Here's how the part is built. I have some questions about the finished solid (model axes, mm). Face numbers are marked on the shaded views. A direction names the side the tool comes from. Round coordinates to 2 decimals unless told otherwise and drop trailing zeros. Order: outer loops, then holes, each group sorted by start corner. A loop starts at its lowest first (then second) coordinate and runs counter-clockwise, first axis right, second up. Notation, with made-up numbers: (41, 41.5) - (62, 41.5) arc R31 cw to (62, 69.5) - close; hole circle Ø10 at (35, -28). An arc over 180 degrees is marked (long way). Answer as a JSON object with one key per item and string values.
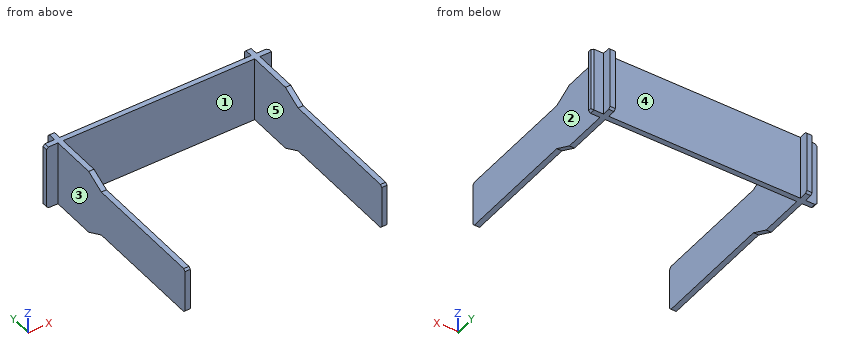
```python
from build123d import *

# Parameters (mm, degrees)
SKETCH1_W           = 2.75
SKETCH1_H           = 5
SKETCH1_W_2         = 6
SKETCH1_H_2         = 2.75
SKETCH1_H_3         = 98.25
SKETCH1_W_3         = 100.5
BOSS_EXTRUDE1_DEPTH = 17
CUT_EXTRUDE1_DEPTH  = 113
CHAMFER1_SIZE       = 1


with BuildPart() as part:
    # Sketch1 → Boss-Extrude1 (new body, symmetric)
    with BuildSketch(Plane.XY):
        with Locations((-51.625, 3.875)):
            Rectangle(SKETCH1_W, SKETCH1_H)
        with Locations((-56, 0)):
            Rectangle(SKETCH1_W_2, SKETCH1_H_2)
        with Locations((-51.625, 0)):
            Rectangle(SKETCH1_W, SKETCH1_H_2)
        with Locations((-51.625, -50.5)):
            Rectangle(SKETCH1_W, SKETCH1_H_3)
        Rectangle(SKETCH1_W_3, SKETCH1_H_2)
        with Locations((51.625, 3.875)):
            Rectangle(SKETCH1_W, SKETCH1_H)
        with Locations((51.625, 0)):
            Rectangle(SKETCH1_W, SKETCH1_H_2)
        with Locations((56, 0)):
            Rectangle(SKETCH1_W_2, SKETCH1_H_2)
        with Locations((51.625, -50.5)):
            Rectangle(SKETCH1_W, SKETCH1_H_3)
    extrude(amount=BOSS_EXTRUDE1_DEPTH, both=True)

    # Sketch2 → Cut-Extrude1 (cut, through all)
    with BuildSketch(Plane(origin=(53, 0, 0), x_dir=(0, 0, -1), z_dir=(1, 0, 0))):
        Polygon((-12, -34.875), (-17, -25.125), (-17, -99.625), (-12, -99.625), align=None)
        Polygon((17, -99.625), (17, -25.125), (12, -34.875), (12, -99.625), align=None)
    extrude(amount=-CUT_EXTRUDE1_DEPTH, mode=Mode.SUBTRACT)

    # Chamfer1
    chamfer1_edges = [part.edges().sort_by_distance(p)[0] for p in [
        (-51.625, 6.375, 17),
        (51.625, -99.625, -12),
        (-59, 0, 17),
        (-51.625, 6.375, -17),
        (51.625, 6.375, -17),
        (59, 0, -17),
        (-59, 0, -17),
        (59, 1.375, 0),
        (51.625, 6.375, 17),
        (-51.625, -99.625, 12),
        (51.625, -99.625, 12),
        (-51.625, -99.625, -12),
    ]]
    chamfer(chamfer1_edges, length=CHAMFER1_SIZE)


solid = part.part
```
1. For the marked faces 4 and 5, which set-ups out of +Z, -Z, +X, -X, +Y, -Y let a thin tool reach every point of the face, with its end or its side?
Responses:
{"face 4": "+Z, -Z, +Y", "face 5": "+Z, -Z, -Y"}
2. If I drill on L1, parallel to X at y = -6, z = -5; L2, parallel to Y at x = 3, z = 14 (3 decimals); L3, parallel to Z at x = 50.5, y = -50.5, over which ranges is the centre line in solid material (lowest first)? Write a range as [from, to].
Responses:
{"L1": "[-53, -50.25], [50.25, 53]", "L2": "[-1.375, 1.375]", "L3": "[-12, 12]"}
3. For P1, Ø1.5, axis at x = 38, z = -5.5, coming from the -Y side (3 decimals); P2, Ø8, axis at y = -73, z = -7.5, coming from the -X side; P3, Ø1.8, axis at x = -55.5, z = -2.5, coming from the +Y side (3 decimals); P4, Ø5.5, axis at y = 3.5, z = -3.5, coming from the -X side, each with a flat end and sliding along its axis, tell me the tip position at first contact or that it passes through.
Responses:
{"P1": "y = -1.375", "P2": "x = -53", "P3": "y = 1.375", "P4": "x = -59"}
4. Thinking about a two-plate mould opening in X: for the marked faces 1, 2 and 3, which applies, pulls with the +X half, pulls with the -X half, needs draft (parallel to the pull), parting line crosses it, or undercut?
Responses:
{"face 1": "undercut", "face 2": "pulls with the +X half", "face 3": "pulls with the -X half"}
5. Imagine slicing it at B-B (z = 0). List the corners of the cut face in (x, y) for me (3 decimals), plus the area to 3 significant figures.
Responses:
{"outline": "(-59, -1.375) - (-53, -1.375) - (-53, -99.625) - (-50.25, -99.625) - (-50.25, -1.375) - (50.25, -1.375) - (50.25, -99.625) - (53, -99.625) - (53, -1.375) - (59, -1.375) - (59, 0.375) - (58, 1.375) - (53, 1.375) - (53, 6.375) - (50.25, 6.375) - (50.25, 1.375) - (-50.25, 1.375) - (-50.25, 6.375) - (-53, 6.375) - (-53, 1.375) - (-59, 1.375) - close", "area": "892 mm2"}
6. Imagine slicing it at A-A (y = -53). List the corners of the cut face in (x, z) for me.
Responses:
{"outline": "(-53, -12) - (-50.25, -12) - (-50.25, 12) - (-53, 12) - close; (50.25, -12) - (53, -12) - (53, 12) - (50.25, 12) - close"}
7. Imagine slicing it at C-C (y = -14). List the corners of the cut face in (x, z) for me.
Responses:
{"outline": "(-53, -17) - (-50.25, -17) - (-50.25, 17) - (-53, 17) - close; (50.25, -17) - (53, -17) - (53, 17) - (50.25, 17) - close"}
8. Imagine slicing it at D-D (x = -19). List the corners of the cut face in (y, z) for me (3 decimals).
Responses:
{"outline": "(-1.375, -17) - (1.375, -17) - (1.375, 17) - (-1.375, 17) - close"}
